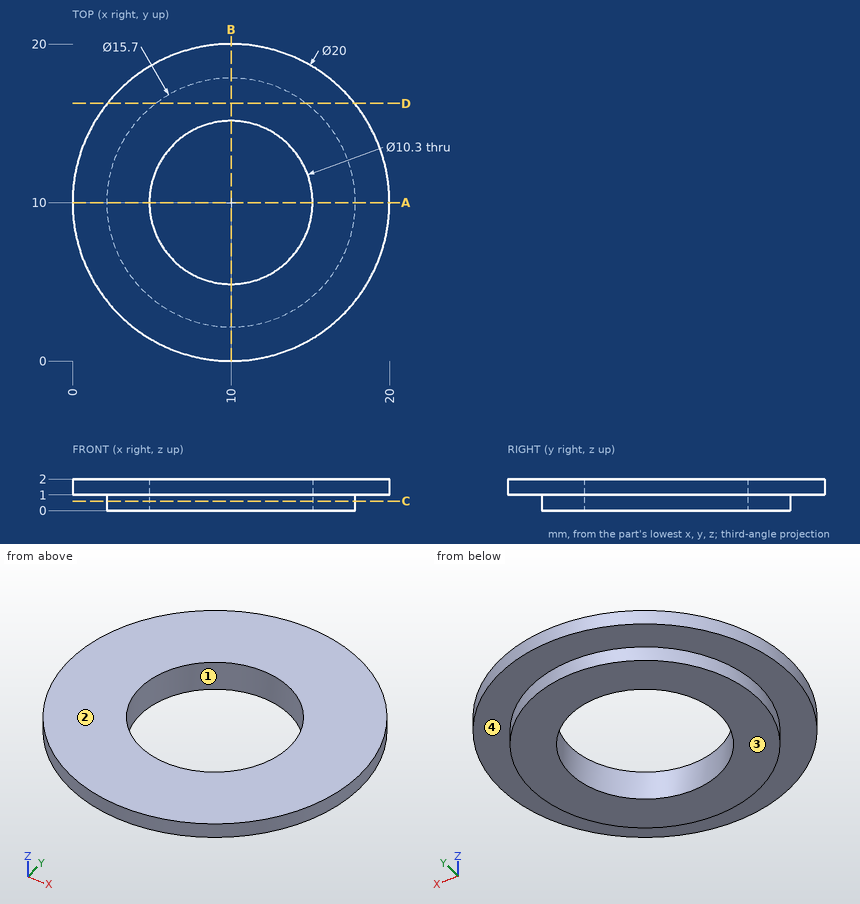
Study the drawing (mm; zero at the part's minimum x, y, z) and answer. A direction names the side the tool comes from. Give positions to 0.01 mm unless a question says otherwise; leave off trailing zeros. Loops run counter-clockwise (first coordinate to the right, second up) from the corner with the lowest first, then second, coordinate; pieces in that order, holes last. Notation, with made-up numbers: (89.5, 61.25) - (119.5, 61.25) arc R30 ccw to (119.5, 85.25) - close; hole circle Ø2 at (-28.5, 38.5). An arc over 180 degrees is marked (long way). Return JSON: item names as keys, results as strings. Group by question number.
1. Find section C-C (z = 0.6). Write down the section's boundary in (x, y).
2. Determine the mould class of the marked faces 1 and 2 for opening direction Y: pulls with the +Y half, pulls with the -Y half, needs draft (parallel to the pull), parting line crosses it, or undercut.
3. Find section A-A (y = 10). Write down the section's boundary in (x, z).
4. Which of the six approach directions +Z, -Z, +X, -X, +Y, -Y give full straight-line access (tool end or side, diameter ignored) to the marked faces 3 and 4?
5. Given pin 1 Ø6 at (x, y) = (10, 10) entering from -Z, flat-ended and moving along its own axis, determine where the tip first touches the part or whether it passes through.
6. Straight lines are drawn through the part: line 1 (Y direction, x = 10, z = 1.55); line 2 (Y direction, x = 10, z = 0.95); line 3 (Z direction, x = 6.25, y = 19). For each, find the intervals that lie inside material, in ascending order. Write a range as [from, to].
7. Find section D-D (y = 16.25). Write down the section's boundary in (x, z), then the cut area to 3 significant figures.
Verdict:
{
 "1": {"outline": "circle Ø15.7 at (10, 10); hole circle Ø10.3 at (10, 10)"},
 "2": {"face 1": "undercut", "face 2": "needs draft"},
 "3": {"outline": "(0, 1) - (2.15, 1) - (2.15, 0) - (4.85, 0) - (4.85, 2) - (0, 2) - close; (15.15, 0) - (17.85, 0) - (17.85, 1) - (20, 1) - (20, 2) - (15.15, 2) - close"},
 "4": {"face 3": "-Z, +X, -X, +Y, -Y", "face 4": "-Z"},
 "5": {"pin 1": "passes through"},
 "6": {"line 1": "y = [0, 4.85], [15.15, 20]", "line 2": "y = [2.15, 4.85], [15.15, 17.85]", "line 3": "z = [1, 2]"},
 "7": {"outline": "(2.19, 1) - (5.25, 1) - (5.25, 0) - (14.75, 0) - (14.75, 1) - (17.81, 1) - (17.81, 2) - (2.19, 2) - close", "area": "25.1 mm^2"}
}
